Autodesk Inventor part; units mm, degrees
ref_plane "YZ Plane" through (0, 0, 0) normal (1, 0, 0) x (0, 1, 0)
ref_plane "XZ Plane" through (0, 0, 0) normal (0, 1, 0) x (-1, 0, 0)
ref_plane "XY Plane" through (0, 0, 0) normal (0, 0, 1) x (1, 0, 0)
sketch "Sketch1" plane through (0, 0, 0) normal (0, 1, 0) x (-1, 0, 0)
  line L0 (0, 0) -> (-20, 0)
  line L1 (-20, 0) -> (-20, -20)
  line L2 (-20, -20) -> (0, -20)
  line L3 (0, -20) -> (0, 0)
  dimension "d0" = 20
  dimension "d1" = 20
extrude "Extrusion1" add sketch "Sketch1" along normal blind 4
sketch "Sketch2" plane through (0, 4, 0) normal (0, 1, 0) x (1, 0, 0)
  line L0 (0, 0) -> (20, 0)
  line L1 (20, 0) -> (20, 4)
  line L2 (20, 4) -> (7, 4)
  line L3 (0, 4) -> (0, 0)
  line L4 (0, 0) -> (4, 0)
  line L5 (7, 20) -> (0, 20)
  line L6 (0, 20) -> (0, 0)
  line L7 (7, 4) -> (7, 20)
  line L8 (0, 0) -> (20, 0)
  line L9 (0, 0) -> (20, 0)
  line L10 (0, 20) -> (0, 0)
  line L11 (0, 0) -> (0, 20)
  dimension "d123" = 7
extrude "Extrusion2" add sketch "Sketch2" along normal blind 45
hole "Hole2" at (12, 12, -4) direction (0, 0, 1) diameter 4 end through all
hole "Hole3" at (7, 12, -12) direction (-1, 0, 0) diameter 4 end through all
hole "Hole4" at (12, 4, -12) direction (0, -1, 0) diameter 4 end through all
sketch "Sketch3" plane through (20, 4, -4) normal (0, 0, -1) x (-1, 0, 0)
  line L0 (12.0415, 8) -> (10.0207, 4.5)
  line L1 (10.0207, 4.5) -> (5.9793, 4.5)
  line L2 (5.9793, 4.5) -> (3.9585, 8)
  line L3 (3.9585, 8) -> (5.9793, 11.5)
  line L4 (5.9793, 11.5) -> (10.0207, 11.5)
  line L5 (10.0207, 11.5) -> (12.0415, 8)
  point P0 (20, -4)
  point P1 (8, 8)
  dimension "d51" = 7
sketch "Sketch4" plane through (7, 4, -4) normal (1, 0, 0) x (0, 0, -1)
  line L0 (12.0415, 8) -> (10.0207, 4.5)
  line L1 (10.0207, 4.5) -> (5.9793, 4.5)
  line L2 (5.9793, 4.5) -> (3.9585, 8)
  line L3 (3.9585, 8) -> (5.9793, 11.5)
  line L4 (5.9793, 11.5) -> (10.0207, 11.5)
  line L5 (10.0207, 11.5) -> (12.0415, 8)
  point P0 (-4, -4)
  point P1 (8, 8)
  dimension "d52" = 7
sketch "Sketch5" plane through (0, 4, 0) normal (0, 1, 0) x (1, 0, 0)
  circle A0 centre (12, 12) radius 2
  line L0 (12, 7.9585) -> (8.5, 9.9793)
  line L1 (8.5, 9.9793) -> (8.5, 14.0207)
  line L2 (8.5, 14.0207) -> (12, 16.0415)
  line L3 (12, 16.0415) -> (15.5, 14.0207)
  line L4 (15.5, 14.0207) -> (15.5, 9.9793)
  line L5 (15.5, 9.9793) -> (12, 7.9585)
  point P0 (0, 0)
  dimension "d53" = 7
extrude "Extrusion3" cut sketch "Sketch3" against normal blind 3.2
extrude "Extrusion4" cut sketch "Sketch4" against normal blind 3.2
extrude "Extrusion5" cut sketch "Sketch5" against normal blind 3.2
sketch "Sketch6" plane through (0, 49, 0) normal (0, 1, 0) x (1, 0, 0)
  line L0 (0, 0) -> (20, 0)
  line L1 (0, 0) -> (0, 46)
  line L2 (0, 20) -> (0, 0)
  line L3 (0, 0) -> (49, 0)
  line L4 (49, 0) -> (49, 14)
  line L5 (0, 46) -> (17, 46)
  line L6 (17, 46) -> (17, 14)
  line L7 (17, 14) -> (49, 14)
  line L8 (20, 4) -> (7, 4)
  line L9 (7, 4) -> (7, 20)
  line L10 (20, 20) -> (7, 20)
  line L11 (20, 4) -> (20, 20)
  line L12 (43.5, 9.5) -> (12.5, 40.5) construction
  line L13 (12.5, 9.5) -> (28, 25) construction
  point P0 (8, 25)
  dimension "d62" = 17
  dimension "d65" = 42
  dimension "d66" = 42
  dimension "d68" = 5.5
  dimension "d69" = 5.5
  dimension "d70" = 31
  dimension "d71" = 31
  dimension "d72" = 14
  dimension "d121" = 8
  dimension "d122" = 25
extrude "Extrusion6" add sketch "Sketch6" along normal blind 6 contours L1 L5 L6 L10 L9 L8 L11 L7 L4 L3 L0 | L11 L8 L9 L10 L6 L7
hole "Hole5" at (12.5, 49, -9.5) at (12.5, 49, -40.5) at (43.5, 49, -9.5) direction (0, 1, 0) diameter 3 end through all
sketch "Sketch7" plane through (0, 55, 0) normal (0, 1, 0) x (1, 0, 0)
  line L0 (0, 0) -> (20, 0)
  line L1 (20, 4) -> (7, 4)
  line L2 (0, 0) -> (20, 0)
  line L3 (20, 0) -> (20, 4)
  line L4 (20, 4) -> (4, 4)
  line L5 (0, 4) -> (0, 0)
  line L6 (0, 0) -> (4, 0)
  line L7 (4, 20) -> (0, 20)
  line L8 (0, 20) -> (0, 0)
  line L9 (4, 4) -> (4, 20)
  dimension "d82" = 20
  dimension "d83" = 4
  dimension "d84" = 4
  dimension "d85" = 20
extrude "Extrusion7" add sketch "Sketch7" along normal blind 16
hole "Hole6" at (12, 63, -4) direction (0, 0, 1) diameter 4 end through all
hole "Hole7" at (4, 63, -12) direction (-1, 0, 0) diameter 4 end through all
sketch "Sketch8" plane through (4, 55, -4) normal (1, 0, 0) x (0, 0, -1)
  line L0 (3.9585, 8) -> (5.9793, 11.5)
  line L1 (5.9793, 11.5) -> (10.0207, 11.5)
  line L2 (10.0207, 11.5) -> (12.0415, 8)
  line L3 (12.0415, 8) -> (10.0207, 4.5)
  line L4 (10.0207, 4.5) -> (5.9793, 4.5)
  line L5 (5.9793, 4.5) -> (3.9585, 8)
  point P0 (-4, -55)
  point P1 (8, 8)
  dimension "d106" = 7
sketch "Sketch9" plane through (20, 55, -4) normal (0, 0, -1) x (-1, 0, 0)
  circle A0 centre (8, 8) radius 2
  line L0 (3.9585, 8) -> (5.9793, 11.5)
  line L1 (5.9793, 11.5) -> (10.0207, 11.5)
  line L2 (10.0207, 11.5) -> (12.0415, 8)
  line L3 (12.0415, 8) -> (10.0207, 4.5)
  line L4 (10.0207, 4.5) -> (5.9793, 4.5)
  line L5 (5.9793, 4.5) -> (3.9585, 8)
  point P0 (20, -55)
  dimension "d107" = 7
extrude "Extrusion8" cut sketch "Sketch9" against normal blind 3.2
extrude "Extrusion9" cut sketch "Sketch8" against normal blind 3.2
hole "Hole8" at (8, 55, -25) direction (0, -1, 0) diameter 8 end through all
sketch "Sketch11" plane through (0, 0, -20) normal (-1, 0, 0) x (0, 0, 1)
  line L0 (0, 0) -> (0, 49)
  line L1 (0, 10.5822) -> (3, 10.5822)
  line L2 (3, 10.5822) -> (3, 21)
  line L3 (3, 21) -> (0, 21)
  line L4 (0, 21) -> (0, 10.5822)
  point P0 (20, 0)
extrude "Extrusion10" cut sketch "Sketch11" against normal blind 10
properties part number "MotorMountLeft" material "PLA Orange"
Can you work these out from the model? Positions are in its coordinate system, mm. A direction names the side the tool comes from. Give positions to 0.01 mm unless a question says otherwise; leave off trailing zeros. Write each loop counter-clockwise with the first axis right and the second up, starting at its lowest first coordinate (ties: lowest second). Pieces come first, ordered by that corner, then holes. Notation, with made-up numbers: M 78,69 L 125,69 A31 cw 125,95 Z; hole C 1,6 d10. An arc over 180 degrees is marked long. Answer in a Markdown table with one row per item. Add a question column.
Item 1: We'd pull the mould along Z, two halves only. Please class faces 4 (the flat face through (8.955, 61.274, -2.422)), 5 (the flat face through (8.5, 2, -12)), 6 (the flat face through (12, 59, -4)): released by +Z, released by -Z, zero draft, split by the parting line, or undercut.
Item 2: On a 3-axis mill with a long thin cutter (end or side, diameter ignored), from which of +Z, -Z, +X, -X, +Y, -Y can I reach the whole of each face in a straight line? I mean faces 1 (the flat face through (14, 26, -4)), 2 (the flat face through (4, 35, -20)), 3 (the flat face through (12, 66.5, -2)). Say none if no direction works.
Item 3: Please list where these lines run through material, in increasing order: L1, parallel to X at y = 51.1, z = -9.5; L2, parallel to Y at x = 0.6, z = -12; L3, parallel to Y at x = 12.5, z = -7.5.
Item 4: Imagine slicing it at C-C, the plane y = 38.5. Write out the boundary of the cut face in (x, z).
Item 5: Imagine slicing it at B-B, the plane x = 43.5. Write out the boundary of the cut face in (y, z).
Item 6: Imagine slicing it at D-D, the plane x = 38. Write out the boundary of the cut face in (y, z), plus the area to 3 significant figures.
Item 7: Imagine slicing it at A-A, the plane z = -25. Write out the boundary of the cut face in (x, y).
Item 8: For pin 1 Ø1.5 at (x, y) = (36.5, 55) entering from -Z; pin 2 Ø4 at (x, z) = (14.5, -9.5) entering from +Y; pin 3 Ø3 at (x, z) = (36, -6.5) entering from -Y, each with a flat end and sliding along its axis, tell me the tip position at first contact or that it passes through.
Evaluation:
| question | item | result |
|---|---|---|
| 1 | face 4 | zero draft |
| 1 | face 5 | undercut |
| 1 | face 6 | released by -Z |
| 2 | face 1 | -Z, +X |
| 2 | face 2 | -Z, +X, -X, -Y |
| 2 | face 3 | -Z |
| 3 | L1 | x = 0 to 11, 14 to 42, 45 to 49 |
| 3 | L2 | y = 0 to 10, 14 to 61, 65 to 71 |
| 3 | L3 | y = 0 to 4, 49 to 55 |
| 4 | outline | M 0,-20 L 7,-20 L 7,-4 L 20,-4 L 20,0 L 0,0 Z |
| 5 | outline | M 49,-14 L 55,-14 L 55,-11 L 49,-11 Z; M 49,-8 L 55,-8 L 55,0 L 49,0 Z |
| 6 | outline | M 49,-14 L 55,-14 L 55,0 L 49,0 Z |
| 6 | area | 84.0 mm² |
| 7 | outline | M 0,49 L 4,49 L 4,55 L 0,55 Z; M 12,49 L 17,49 L 17,55 L 12,55 Z |
| 8 | pin 1 | stops at z = -14 |
| 8 | pin 2 | stops at y = 55 |
| 8 | pin 3 | stops at y = 49 |
